from build123d import *

# Parameters (mm, degrees)
CYLINDER022_R             = 0.95
CYLINDER022_DEPTH         = 10
CYLINDER023_R             = 0.95
CYLINDER023_DEPTH         = 10
CYLINDER020_R             = 0.95
CYLINDER020_DEPTH         = 10
CYLINDER021_R             = 0.95
CYLINDER021_DEPTH         = 10
BOX004_W                  = 10
BOX004_H                  = 10
BOX004_DEPTH              = 7
PAD007_DEPTH              = 21
CYLINDER019_R             = 3
CYLINDER019_DEPTH         = 10
CYLINDER027_R             = 0.95
CYLINDER027_DEPTH         = 10
CYLINDER028_R             = 0.95
CYLINDER028_DEPTH         = 10
CYLINDER025_R             = 0.95
CYLINDER025_DEPTH         = 10
CYLINDER026_R             = 0.95
CYLINDER026_DEPTH         = 10
BOX005_W                  = 10
BOX005_H                  = 10
BOX005_DEPTH              = 7
PAD008_DEPTH              = 21
CYLINDER024_R             = 3
CYLINDER024_DEPTH         = 10
FUSION022_PLACEMENT_ANGLE = 180


with BuildPart() as cylinder022:
    # Cylinder022 → Cylinder022 (new body)
    with BuildSketch(Plane(origin=(9.9, 0, 0), x_dir=(1, 0, 0), z_dir=(0, 0, 1))):
        Circle(CYLINDER022_R)
    extrude(amount=CYLINDER022_DEPTH)


with BuildPart() as tornillos009:
    # Cylinder023 → Cylinder023 (new body)
    with BuildSketch(Plane.XY):
        Circle(CYLINDER023_R)
    extrude(amount=CYLINDER023_DEPTH)

    # Fusion016: union Cylinder022
    add(cylinder022.part)


with BuildPart() as tornillos009_1:
    # Fusion016 placement: moved
    add(tornillos009.part.moved(Location((5, -24.5, 22))))


with BuildPart() as cylinder020:
    # Cylinder020 → Cylinder020 (new body)
    with BuildSketch(Plane(origin=(9.9, 0, 0), x_dir=(1, 0, 0), z_dir=(0, 0, 1))):
        Circle(CYLINDER020_R)
    extrude(amount=CYLINDER020_DEPTH)


with BuildPart() as fusion017:
    # Cylinder021 → Cylinder021 (new body)
    with BuildSketch(Plane.XY):
        Circle(CYLINDER021_R)
    extrude(amount=CYLINDER021_DEPTH)

    # Fusion015: union Cylinder020
    add(cylinder020.part)


with BuildPart() as fusion017_1:
    # Fusion015 placement: moved
    add(fusion017.part.moved(Location((5, 24.5, 22))))

    # Fusion017: union Tornillos009
    add(tornillos009_1.part)


with BuildPart() as fusion017_2:
    # Fusion017 placement: moved
    add(fusion017_1.part.moved(Location((0.4, 0, 0))))


with BuildPart() as cube004:
    # Box004 → Box004 (new body)
    with BuildSketch(Plane(origin=(5, -29, 7), x_dir=(1, 0, 0), z_dir=(0, 0, 1))):
        with Locations((5, 5)):
            Rectangle(BOX004_W, BOX004_H)
    extrude(amount=BOX004_DEPTH)


with BuildPart() as holder005:
    # Sketch007 → Pad007 (new body)
    with BuildSketch(Plane.YZ):
        Polygon((-28.75, 32), (-28.75, 0), (28.75, 0), (28.75, 32), (20.75, 32), (20.75, 3.5), (-20.75, 3.5), (-20.75, 32), align=None)
    extrude(amount=PAD007_DEPTH)

    # Cut010: cut Cube004
    add(cube004.part, mode=Mode.SUBTRACT)

    # Cut011: cut Fusion017
    add(fusion017_2.part, mode=Mode.SUBTRACT)


with BuildPart() as obj1:
    # Cylinder019 → Cylinder019 (new body)
    with BuildSketch(Plane(origin=(10.5, -10.1, -7), x_dir=(1, 0, 0), z_dir=(0, 0, 1))):
        Circle(CYLINDER019_R)
    extrude(amount=CYLINDER019_DEPTH)

    # Fusion018: union Holder005
    add(holder005.part)


with BuildPart() as cylinder027:
    # Cylinder027 → Cylinder027 (new body)
    with BuildSketch(Plane(origin=(9.9, 0, 0), x_dir=(1, 0, 0), z_dir=(0, 0, 1))):
        Circle(CYLINDER027_R)
    extrude(amount=CYLINDER027_DEPTH)


with BuildPart() as tornillos011:
    # Cylinder028 → Cylinder028 (new body)
    with BuildSketch(Plane.XY):
        Circle(CYLINDER028_R)
    extrude(amount=CYLINDER028_DEPTH)

    # Fusion020: union Cylinder027
    add(cylinder027.part)


with BuildPart() as tornillos011_1:
    # Fusion020 placement: moved
    add(tornillos011.part.moved(Location((5, -24.5, 22))))


with BuildPart() as cylinder025:
    # Cylinder025 → Cylinder025 (new body)
    with BuildSketch(Plane(origin=(9.9, 0, 0), x_dir=(1, 0, 0), z_dir=(0, 0, 1))):
        Circle(CYLINDER025_R)
    extrude(amount=CYLINDER025_DEPTH)


with BuildPart() as fusion021:
    # Cylinder026 → Cylinder026 (new body)
    with BuildSketch(Plane.XY):
        Circle(CYLINDER026_R)
    extrude(amount=CYLINDER026_DEPTH)

    # Fusion019: union Cylinder025
    add(cylinder025.part)


with BuildPart() as fusion021_1:
    # Fusion019 placement: moved
    add(fusion021.part.moved(Location((5, 24.5, 22))))

    # Fusion021: union Tornillos011
    add(tornillos011_1.part)


with BuildPart() as fusion021_2:
    # Fusion021 placement: moved
    add(fusion021_1.part.moved(Location((0.4, 0, 0))))


with BuildPart() as cube005:
    # Box005 → Box005 (new body)
    with BuildSketch(Plane(origin=(5, -29, 7), x_dir=(1, 0, 0), z_dir=(0, 0, 1))):
        with Locations((5, 5)):
            Rectangle(BOX005_W, BOX005_H)
    extrude(amount=BOX005_DEPTH)


with BuildPart() as holder006:
    # Sketch008 → Pad008 (new body)
    with BuildSketch(Plane.YZ):
        Polygon((-28.75, 32), (-28.75, 0), (28.75, 0), (28.75, 32), (20.75, 32), (20.75, 3.5), (-20.75, 3.5), (-20.75, 32), align=None)
    extrude(amount=PAD008_DEPTH)

    # Cut012: cut Cube005
    add(cube005.part, mode=Mode.SUBTRACT)

    # Cut013: cut Fusion021
    add(fusion021_2.part, mode=Mode.SUBTRACT)


with BuildPart() as fusion023:
    # Cylinder024 → Cylinder024 (new body)
    with BuildSketch(Plane(origin=(10.5, -10.1, -7), x_dir=(1, 0, 0), z_dir=(0, 0, 1))):
        Circle(CYLINDER024_R)
    extrude(amount=CYLINDER024_DEPTH)

    # Fusion022: union Holder006
    add(holder006.part)


with BuildPart() as fusion023_1:
    # Fusion022 placement: moved
    add(fusion023.part.moved(Location((21, 57, 0))).rotate(Axis((21, 57, 0), (0, 0, 1)), FUSION022_PLACEMENT_ANGLE))

    # Fusion023: union obj1
    add(obj1.part)


solid = fusion023_1.part
Can you work these out from the model? Positions are in its coordinate system, mm. A direction names the side the tool comes from. Give positions to 0.01 mm unless a question says otherwise; leave off trailing zeros. Loops run counter-clockwise (first coordinate to the right, second up) from the corner with the lowest first, then second, coordinate; pieces in that order, holes last. Notation, with made-up numbers: (50, 25) -> (84, 25) arc R31 cw to (84, 59) -> close; hole circle Ø1 at (-14, 88). An arc over 180 degrees is marked (long way). Write item = value, one per line.
1) For faces 1 (the cylindrical face through (5.194, 23.573, 26.93)), 2 (the flat face through (11, 82, 7)), 3 (the cylindrical face through (8.29, -8.07, -3.55)), 4 (the flat face through (5, -25, 10)), 5 (the flat face through (10, -10, -7)), which set-ups out of +Z, -Z, +X, -X, +Y, -Y let a thin tool reach every point of the face, with its end or its side?
Check result:
face_1 = +Z
face_2 = +Y
face_3 = -Z
face_4 = -Y
face_5 = -Z, +X, -X, +Y, -Y
2) Suppose I cut it at A-A on z = 30. Give the number of separate pieces and of enclosed holes in the cut face, then the cut area to 3 significant figures.
Check result:
separate_pieces = 3
enclosed_holes = 8
area = 639 mm2
3) Will these pins go through, and if not, where does the flat tip stop? pin 1 (6 mm diameter, centred on x = 9.5, y = 23, fed in from -Z); pin 2 (0.9 mm diameter, centred on x = 15.5, y = 24.5, fed in from +Z); pin 3 (10 mm diameter, centred on x = 18.5, y = 71.5, fed in from +Z); pin 4 (10 mm diameter, centred on y = 54, z = 9, fed in from -X).
Check result:
pin_1 = 0
pin_2 = 22
pin_3 = 3.5
pin_4 = through
4) Suppose I cut it at D-D on z = -3.5. Write out the boundary of the cut face in (x, y).
Check result:
outline = circle Ø6 at (10.5, -10.1); circle Ø6 at (10.5, 67.1)
5) Suppose I cut it at C-C on y = -10.1. Write out the boundary of the cut face in (x, z), then the cut area to 4 significant figures.
Check result:
outline = (0, 0) -> (7.5, 0) -> (7.5, -7) -> (13.5, -7) -> (13.5, 0) -> (21, 0) -> (21, 3.5) -> (0, 3.5) -> close
area = 115.5 mm2
6) Suppose I cut it at B-B on z = 13. Write out the boundary of the cut face in (x, y).
Check result:
outline = (0, -28.75) -> (5, -28.75) -> (5, -20.75) -> (0, -20.75) -> close; (0, 20.75) -> (21, 20.75) -> (21, 36.25) -> (0, 36.25) -> close; (0, 77.75) -> (6, 77.75) -> (6, 85.75) -> (0, 85.75) -> close; (15, -28.75) -> (21, -28.75) -> (21, -20.75) -> (15, -20.75) -> close; (16, 77.75) -> (21, 77.75) -> (21, 85.75) -> (16, 85.75) -> close
7) Thinking about a two-plate mould opening in Z: for faces 6 (the flat face through (10, -25, 7)), 7 (the flat face through (11, 67, -7)), 8 (the flat face through (11, 77.75, 18)), which applies, released by +Z, released by -Z, zero draft, split by the parting line, or undercut?
Check result:
face_6 = undercut
face_7 = released by -Z
face_8 = zero draft
8) I need wall thicknesses on L1, parallel to Y at x = 11, z = 30; L2, parallel to X at y = 32.5, z = 29.25; L3, parallel to X at y = -24, z = 26. Which ranges of each line are inside material? Lowest first, please. Write a range as from..to.
Check result:
L1 = -28.75..-20.75, 20.75..36.25, 77.75..85.75
L2 = 0..4.75, 6.65..14.65, 16.55..21
L3 = 0..4.59, 6.21..14.49, 16.11..21
